```python
from build123d import *

# Parameters (mm, degrees)
SKETCH1_W            = 56
SKETCH1_H            = 32
SKETCH1_W_2          = 50
SKETCH1_H_2          = 26
BOSS_EXTRUDE1_DEPTH  = 3
SKETCH2_W            = 3
SKETCH2_H            = 3
BOSS_EXTRUDE2_DEPTH  = 40
BOSS_EXTRUDE3_DEPTH  = 3
BOSS_EXTRUDE4_DEPTH  = 3
SKETCH5_W            = 3
SKETCH5_H            = 26
BOSS_EXTRUDE5_DEPTH  = 3
SKETCH6_W            = 50
SKETCH6_H            = 3
SKETCH6_W_2          = 3
BOSS_EXTRUDE7_DEPTH  = 3
SKETCH7_W            = 3
SKETCH7_H            = 3
BOSS_EXTRUDE8_DEPTH  = 15
SKETCH8_W            = 3
SKETCH8_H            = 26
SKETCH8_W_2          = 6
SKETCH8_H_2          = 3
BOSS_EXTRUDE9_DEPTH  = 3
BOSS_EXTRUDE10_DEPTH = 3
BOSS_EXTRUDE11_DEPTH = 3


with BuildPart() as part:
    # Sketch1 → Boss-Extrude1 (new body)
    with BuildSketch(Plane(origin=(0, 0, 0), x_dir=(1, 0, 0), z_dir=(0, 1, 0))):
        Rectangle(SKETCH1_W, SKETCH1_H)
        Rectangle(SKETCH1_W_2, SKETCH1_H_2, mode=Mode.SUBTRACT)
    extrude(amount=BOSS_EXTRUDE1_DEPTH)

    # Sketch2 → Boss-Extrude2 (add)
    with BuildSketch(Plane(origin=(0, 0, 0), x_dir=(1, 0, 0), z_dir=(0, 1, 0))):
        with Locations((26.5, 14.5)):
            Rectangle(SKETCH2_W, SKETCH2_H)
        with Locations((26.5, -14.5)):
            Rectangle(SKETCH2_W, SKETCH2_H)
        with Locations((-26.5, -14.5)):
            Rectangle(SKETCH2_W, SKETCH2_H)
        with Locations((-26.5, 14.5)):
            Rectangle(SKETCH2_W, SKETCH2_H)
    extrude(amount=BOSS_EXTRUDE2_DEPTH)

    # Sketch3 → Boss-Extrude3 (add)
    with BuildSketch(Plane.XY.offset(16)):
        Polygon((28, 10), (28, 5), (29.7, 5), (29.7, 8.2), (32.9, 8.2), (32.9, 6.6), (36.1, 6.6), (36.1, 5), (38, 5), (38, 10), align=None)
        Polygon((28, 5), (28, 0), (38, 0), (38, 5), (36.1, 5), (36.1, 3.4), (32.9, 3.4), (32.9, 1.8), (29.7, 1.8), (29.7, 5), align=None)
    boss_extrude3 = extrude(amount=-BOSS_EXTRUDE3_DEPTH)

    # Mirror1: Boss-Extrude3 across plane
    add(boss_extrude3.mirror(Plane.XY))

    # Sketch4 → Boss-Extrude4 (add)
    with BuildSketch(Plane.XY.offset(16)):
        Polygon((5, 0), (0, 0), (-5, 0), (-5, -10), (0, -10), (5, -10), align=None)
        Polygon((1.6, -8.1), (0, -8.1), (-1.6, -8.1), (-1.6, -4.9), (-3.2, -4.9), (-3.2, -1.7), (3.2, -1.7), (3.2, -4.9), (1.6, -4.9), align=None, mode=Mode.SUBTRACT)
    boss_extrude4 = extrude(amount=-BOSS_EXTRUDE4_DEPTH)

    # Mirror2: Boss-Extrude4 across plane
    add(boss_extrude4.mirror(Plane.XY))

    # Sketch5 → Boss-Extrude5 (add)
    with BuildSketch(Plane(origin=(0, 3, 0), x_dir=(1, 0, 0), z_dir=(0, 1, 0))):
        with Locations((-17, 0)):
            Rectangle(SKETCH5_W, SKETCH5_H)
        with Locations((-8, 0)):
            Rectangle(SKETCH5_W, SKETCH5_H)
        with Locations((8, 0)):
            Rectangle(SKETCH5_W, SKETCH5_H)
        with Locations((17, 0)):
            Rectangle(SKETCH5_W, SKETCH5_H)
    extrude(amount=-BOSS_EXTRUDE5_DEPTH)

    # Sketch6 → Boss-Extrude7 (add)
    # profile 1 of 4: a face of its own
    with BuildSketch(Plane(origin=(0, 40, 0), x_dir=(1, 0, 0), z_dir=(0, 1, 0))):
        Polygon((-28, -16), (25, -16), (25, -13), (28, -13), (28, 16), (-28, 16), align=None)
        Polygon((25, -9), (25, -13), (-25, -13), (-25, -9), (-25, -6), (-25, 6), (-25, 9), (-25, 13), (25, 13), (25, 9), (25, 6), (25, -6), align=None, mode=Mode.SUBTRACT)
    # profile 2 of 4: a face of its own
    with BuildSketch(Plane(origin=(0, 40, 0), x_dir=(1, 0, 0), z_dir=(0, 1, 0))):
        with Locations((0, -7.5)):
            Rectangle(SKETCH6_W, SKETCH6_H)
    # profile 3 of 4: a face of its own
    with BuildSketch(Plane(origin=(0, 40, 0), x_dir=(1, 0, 0), z_dir=(0, 1, 0))):
        with Locations((0, 7.5)):
            Rectangle(SKETCH6_W, SKETCH6_H)
    # profile 4 of 4: a face of its own
    with BuildSketch(Plane(origin=(0, 40, 0), x_dir=(1, 0, 0), z_dir=(0, 1, 0))):
        with Locations((26.5, -14.5)):
            Rectangle(SKETCH6_W_2, SKETCH6_H)
    extrude(amount=BOSS_EXTRUDE7_DEPTH)

    # Sketch7 → Boss-Extrude8 (add)
    with BuildSketch(Plane(origin=(0, 43, 0), x_dir=(1, 0, 0), z_dir=(0, 1, 0))):
        with Locations((-26.5, -14.5)):
            Rectangle(SKETCH7_W, SKETCH7_H)
        with Locations((-26.5, 14.5)):
            Rectangle(SKETCH7_W, SKETCH7_H)
        with Locations((26.5, 14.5)):
            Rectangle(SKETCH7_W, SKETCH7_H)
        with Locations((26.5, -14.5)):
            Rectangle(SKETCH7_W, SKETCH7_H)
    extrude(amount=BOSS_EXTRUDE8_DEPTH)

    # Sketch8 → Boss-Extrude9 (add)
    # profile 1 of 5: a face of its own
    with BuildSketch(Plane(origin=(0, 58, 0), x_dir=(1, 0, 0), z_dir=(0, 1, 0))):
        Polygon((-25, 16), (-25, 13), (-28, 13), (-28, -16), (28, -16), (28, 16), align=None)
        Polygon((25, 13), (25, -13), (15.5, -13), (12.5, -13), (9.5, -13), (0, -13), (-9.5, -13), (-15.5, -13), (-25, -13), (-25, 13), (-15.5, 13), (-9.5, 13), (9.5, 13), (12.5, 13), (15.5, 13), align=None, mode=Mode.SUBTRACT)
    # profile 2 of 5: a face of its own
    with BuildSketch(Plane(origin=(0, 58, 0), x_dir=(1, 0, 0), z_dir=(0, 1, 0))):
        with Locations((11, 0)):
            Rectangle(SKETCH8_W, SKETCH8_H)
    # profile 3 of 5: a face of its own
    with BuildSketch(Plane(origin=(0, 58, 0), x_dir=(1, 0, 0), z_dir=(0, 1, 0))):
        with Locations((14, 0)):
            Rectangle(SKETCH8_W, SKETCH8_H)
    # profile 4 of 5: a face of its own
    with BuildSketch(Plane(origin=(0, 58, 0), x_dir=(1, 0, 0), z_dir=(0, 1, 0))):
        with Locations((-12.5, 0)):
            Rectangle(SKETCH8_W_2, SKETCH8_H)
    # profile 5 of 5: a face of its own
    with BuildSketch(Plane(origin=(0, 58, 0), x_dir=(1, 0, 0), z_dir=(0, 1, 0))):
        with Locations((-26.5, 14.5)):
            Rectangle(SKETCH8_W, SKETCH8_H_2)
    extrude(amount=BOSS_EXTRUDE9_DEPTH)

    # Sketch9 → Boss-Extrude10 (add)
    with BuildSketch(Plane.XZ.offset(10)):
        with BuildLine():
            ThreePointArc((-5, -5.25), (-3.378132989, -6.414882502), (-1.5, -7.09313048))
            Line((-1.5, -7.09313048), (-1.5, -4.083197277))
            ThreePointArc((-1.5, -4.083197277), (-4.35, 0), (-1.5, 4.083197277))
            Line((-1.5, 4.083197277), (-1.5, 7.09313048))
            ThreePointArc((-1.5, 7.09313048), (-3.378132989, 6.414882502), (-5, 5.25))
            Line((-5, 5.25), (-5, -5.25))
        make_face()
        with BuildLine():
            ThreePointArc((-5, 5.25), (-7.25, 0), (-5, -5.25))
            Line((-5, -5.25), (-5, 5.25))
        make_face()
        with BuildLine():
            Line((-1.5, -4.083197277), (-1.5, -7.09313048))
            ThreePointArc((-1.5, -7.09313048), (-0.051031089, -7.2498204), (1.4, -7.113543421))
            Line((1.4, -7.113543421), (1.4, -4.118555572))
            ThreePointArc((1.4, -4.118555572), (-0.053033501, -4.349676706), (-1.5, -4.083197277))
        make_face()
        with BuildLine():
            Line((-1.5, 7.09313048), (-1.5, 4.083197277))
            ThreePointArc((-1.5, 4.083197277), (-0.053033501, 4.349676706), (1.4, 4.118555572))
            Line((1.4, 4.118555572), (1.4, 7.113543421))
            ThreePointArc((1.4, 7.113543421), (-0.051031089, 7.2498204), (-1.5, 7.09313048))
        make_face()
        with BuildLine():
            Line((1.4, -4.118555572), (1.4, -7.113543421))
            ThreePointArc((1.4, -7.113543421), (3.332896416, -6.438501493), (5, -5.25))
            Line((5, -5.25), (5, 5.25))
            ThreePointArc((5, 5.25), (3.332896416, 6.438501493), (1.4, 7.113543421))
            Line((1.4, 7.113543421), (1.4, 4.118555572))
            ThreePointArc((1.4, 4.118555572), (3.536417679, 2.53303178), (4.35, 0))
            ThreePointArc((4.35, 0), (3.536417679, -2.53303178), (1.4, -4.118555572))
        make_face()
        with BuildLine():
            Line((5, 5.25), (5, -5.25))
            ThreePointArc((5, -5.25), (6.663801468, -2.855914915), (7.25, 0))
            ThreePointArc((7.25, 0), (6.663801468, 2.855914915), (5, 5.25))
        make_face()
        with BuildLine():
            Line((-1.5, 13), (-1.5, 7.09313048))
            ThreePointArc((-1.5, 7.09313048), (-0.051031089, 7.2498204), (1.4, 7.113543421))
            Line((1.4, 7.113543421), (1.4, 13))
            Line((1.4, 13), (-1.5, 13))
        make_face()
        Polygon((-5, 16), (-5, 13), (-1.5, 13), (1.4, 13), (5, 13), (5, 16), align=None)
        with BuildLine():
            Line((-1.5, -13), (0, -13))
            Line((0, -13), (1.4, -13))
            Line((1.4, -13), (1.4, -7.113543421))
            ThreePointArc((1.4, -7.113543421), (-0.051031089, -7.2498204), (-1.5, -7.09313048))
            Line((-1.5, -7.09313048), (-1.5, -13))
        make_face()
        Polygon((1.4, -13), (0, -13), (-1.5, -13), (-5, -13), (-5, -16), (5, -16), (5, -13), align=None)
    extrude(amount=BOSS_EXTRUDE10_DEPTH)

    # Sketch10 → Boss-Extrude11 (add)
    with BuildSketch(Plane(origin=(28, 0, 0), x_dir=(0, 0, -1), z_dir=(1, 0, 0))):
        Polygon((5, 0), (0, 0), (-5, 0), (-5, -10), (0, -10), (5, -10), align=None)
        Polygon((1.6, -8.1), (0, -8.1), (-1.6, -8.1), (-1.6, -4.9), (-3.1, -4.9), (-3.1, -1.7), (3.1, -1.7), (3.1, -4.9), (1.6, -4.9), align=None, mode=Mode.SUBTRACT)
    boss_extrude11 = extrude(amount=-BOSS_EXTRUDE11_DEPTH)

    # Mirror3: Boss-Extrude11 across plane
    add(boss_extrude11.mirror(Plane(origin=(0, 0, 0), x_dir=(0, 0, 1), z_dir=(1, 0, 0))))


solid = part.part
```
Source: CAD feature listing. Evaluate the final solid. Frame: model axes, mm. A direction names the side the tool comes from. Coordinates: 2 decimals unless noted, no trailing zeros. Loops run counter-clockwise (first coordinate to the right, second up) from the corner with the lowest first, then second, coordinate; pieces in that order, holes last. Notation, with made-up numbers: M 83,84 L 126,84 A23 ccw 126,120 Z; hole C -3.75,-18.5 d10. An arc over 180 degrees is marked long. Put each result on its own line as item: value. Start each with the question number.
1) Cut plane C-C on x = -23.5. Give the number of separate pieces and of enclosed holes in the cut face, then the cut area to 3 significant figures.
2) Cut plane A-A on y = 14.5. Return the cut outline in (x, z), then the cut area to 3 significant figures.
3) Cut plane B-B on x = -12.5. Return the cut outline in (y, z), then the cut area to 3 significant figures.
4) Reachability of faces 1 (the face through (27.6, 15.6, -13)), 2 (the face through (-27, 58, 0)), 3 (the face through (0, -1, 13)), 4 (the face through (-1.6, -7, -15)) from +Z, -Z, +X, -X, +Y, -Y: full face, straight path, thin tool, end or side. Return the list, or none.
5) Pull-direction query (Y, two-part tool) for faces 5 (the face through (-25, 41, 11)), 6 (the face through (-25, 50, -14)); classes: pulls with the +Y half, pulls with the -Y half, needs draft (parallel to the pull), parting line crosses it, or undercut.
6) Contact query for flat-ended pins moving along their axis: pin 1 Ø2.5 at (y, z) = (-8, 15) entering from +X; pin 2 Ø0.9 at (y, z) = (2, 1) entering from +X; pin 3 Ø11.5 at (x, z) = (1, -4.5) entering from +Y. Output: stop coordinate, or through.
7) Ray query, L1, parallel to X at y = 1.5, z = 8; L2, parallel to Z at x = 2.5, y = 2.5; L3, parallel to Z at x = -24.5, y = 41.5. Return the intervals inside material, ascending. Write a range as from..to.
The answers:
1. separate pieces: 8
1. enclosed holes: 0
1. area: 72.0 mm²
2. outline: M -28,-16 L -25,-16 L -25,-13 L -28,-13 Z; M -28,13 L -25,13 L -25,16 L -28,16 Z; M 25,-16 L 28,-16 L 28,-13 L 25,-13 Z; M 25,13 L 28,13 L 28,16 L 25,16 Z
2. area: 36.0 mm²
3. outline: M 0,-16 L 3,-16 L 3,-13 L 0,-13 Z; M 0,13 L 3,13 L 3,16 L 0,16 Z; M 40,-16 L 43,-16 L 43,-13 L 40,-13 Z; M 40,-9 L 43,-9 L 43,-6 L 40,-6 Z; M 40,6 L 43,6 L 43,9 L 40,9 Z; M 40,13 L 43,13 L 43,16 L 40,16 Z; M 58,-16 L 61,-16 L 61,16 L 58,16 Z
3. area: 150 mm²
4. face 1: +X
4. face 2: +X, -X
4. face 3: +Y
4. face 4: +Z, -Z
5. face 5: needs draft
5. face 6: undercut
6. pin 1: stops at x = 5
6. pin 2: stops at x = 28
6. pin 3: stops at y = 43
7. L1: x = -28..-25, -18.5..-15.5, -9.5..-6.5, 6.5..9.5, 15.5..18.5, 25..28
7. L2: z = -16..-13, 13..16
7. L3: z = -16..-13, -9..-6, 6..9, 13..16
